Source: CAD feature listing. Evaluate the final solid. Frame: model axes, mm. Give positions to 0.01 mm unless a question says otherwise; leave off trailing zeros. Write each loop counter-clockwise with the first axis right and the second up, starting at its lowest first coordinate (ties: lowest second). Pieces come first, ordered by that corner, then holes. Notation, with made-up numbers: (34.25, 60) - (55.25, 60) arc R20 ccw to (55.25, 68) - close; hole circle Ø4 at (15, -37). An arc over 180 degrees is marked (long way). Answer as a JSON object with one key per item and string values. Group by question number.
from build123d import *

# Parameters (mm, degrees)
SKETCH1_W           = 304.8
SKETCH1_H           = 50.8
SKETCH1_W_2         = 5.9944
SKETCH1_H_2         = 12.7
BOSS_EXTRUDE1_DEPTH = 5.9944
SKETCH3_W           = 247.65
SKETCH3_H           = 1.4875
CUT_EXTRUDE3_DEPTH  = 6.9944
FILLET4_R           = 0.7
SKETCH4_W           = 28.575
SKETCH4_H           = 50.8
BOSS_EXTRUDE2_DEPTH = 5.9944
SKETCH5_W           = 5.9944
SKETCH5_H           = 12.7
CUT_EXTRUDE4_DEPTH  = 6.9944
FILLET5_R           = 3.175
CUT_EXTRUDE5_DEPTH  = 6.9944
CUT_EXTRUDE6_DEPTH  = 6.9944


with BuildPart() as part:
    # Sketch1 → Boss-Extrude1 (new body)
    with BuildSketch(Plane.XY):
        with Locations((-152.4, 25.4)):
            Rectangle(SKETCH1_W, SKETCH1_H)
        with Locations((-15.6972, 12.7)):
            Rectangle(SKETCH1_W_2, SKETCH1_H_2, mode=Mode.SUBTRACT)
        with Locations((-15.6972, 38.1)):
            Rectangle(SKETCH1_W_2, SKETCH1_H_2, mode=Mode.SUBTRACT)
        with Locations((-257.3528, 38.1)):
            Rectangle(SKETCH1_W_2, SKETCH1_H_2, mode=Mode.SUBTRACT)
        with Locations((-257.3528, 12.7)):
            Rectangle(SKETCH1_W_2, SKETCH1_H_2, mode=Mode.SUBTRACT)
        with Locations((-295.4528, 12.7)):
            Rectangle(SKETCH1_W_2, SKETCH1_H_2, mode=Mode.SUBTRACT)
        with Locations((-295.4528, 38.1)):
            Rectangle(SKETCH1_W_2, SKETCH1_H_2, mode=Mode.SUBTRACT)
    extrude(amount=BOSS_EXTRUDE1_DEPTH)

    # Sketch3 → Cut-Extrude3 (cut, through all)
    with BuildSketch(Plane.XY.offset(5.9944)):
        with Locations((-136.525, 50.05625)):
            Rectangle(SKETCH3_W, SKETCH3_H)
        with Locations((-136.525, 0.74375)):
            Rectangle(SKETCH3_W, SKETCH3_H)
    extrude(amount=-CUT_EXTRUDE3_DEPTH, mode=Mode.SUBTRACT)

    # Fillet4
    fillet4_edges = [part.edges().sort_by_distance(p)[0] for p in [
        (-260.35, 49.3125, 2.9972),
        (-260.35, 50.8, 2.9972),
        (-12.7, 50.8, 2.9972),
        (-12.7, 49.3125, 2.9972),
        (-12.7, 0, 2.9972),
        (-260.35, 0, 2.9972),
        (-260.35, 1.4875, 2.9972),
        (-12.7, 1.4875, 2.9972),
    ]]
    fillet(fillet4_edges, radius=FILLET4_R)

    # Sketch4 → Boss-Extrude2 (add)
    with BuildSketch(Plane.XY.offset(5.9944)):
        with Locations((14.2875, 25.4)):
            Rectangle(SKETCH4_W, SKETCH4_H)
    extrude(amount=-BOSS_EXTRUDE2_DEPTH)

    # Sketch5 → Cut-Extrude4 (cut, through all)
    with BuildSketch(Plane.XY.offset(5.9944)):
        with Locations((21.893276, 38.1)):
            Rectangle(SKETCH5_W, SKETCH5_H)
        with Locations((21.893276, 12.7)):
            Rectangle(SKETCH5_W, SKETCH5_H)
    extrude(amount=-CUT_EXTRUDE4_DEPTH, mode=Mode.SUBTRACT)

    # Fillet5
    fillet5_edges = [part.edges().sort_by_distance(p)[0] for p in [
        (28.575, 50.8, 2.9972),
        (28.575, 0, 2.9972),
        (-304.8, 0, 2.9972),
        (-304.8, 50.8, 2.9972),
    ]]
    fillet(fillet5_edges, radius=FILLET5_R)

    # Sketch6 → Cut-Extrude5 (cut, through all)
    with BuildSketch(Plane.XY.offset(5.9944)):
        with BuildLine():
            Line((-123.825, 19.05), (-149.225, 19.05))
            ThreePointArc((-149.225, 19.05), (-155.575, 25.4), (-149.225, 31.75))
            Line((-149.225, 31.75), (-123.825, 31.75))
            ThreePointArc((-123.825, 31.75), (-117.475, 25.4), (-123.825, 19.05))
        make_face()
        with BuildLine():
            Line((-60.325, 19.05), (-85.725, 19.05))
            ThreePointArc((-85.725, 19.05), (-92.075, 25.4), (-85.725, 31.75))
            Line((-85.725, 31.75), (-60.325, 31.75))
            ThreePointArc((-60.325, 31.75), (-53.975, 25.4), (-60.325, 19.05))
        make_face()
        with BuildLine():
            Line((-187.325, 19.05), (-212.725, 19.05))
            ThreePointArc((-212.725, 19.05), (-219.075, 25.4), (-212.725, 31.75))
            Line((-212.725, 31.75), (-187.325, 31.75))
            ThreePointArc((-187.325, 31.75), (-180.975, 25.4), (-187.325, 19.05))
        make_face()
    extrude(amount=-CUT_EXTRUDE5_DEPTH, mode=Mode.SUBTRACT)

    # Sketch7 → Cut-Extrude6 (cut, through all)
    with BuildSketch(Plane.XY.offset(5.9944)):
        with BuildLine():
            Line((-6.35, 12.7), (-6.35, 38.1))
            ThreePointArc((-6.35, 38.1), (-4.7625, 39.6875), (-3.175, 38.1))
            Line((-3.175, 38.1), (-3.175, 12.7))
            ThreePointArc((-3.175, 12.7), (-4.7625, 11.1125), (-6.35, 12.7))
        make_face()
        with BuildLine():
            Line((1.524, 12.7), (1.524, 38.1))
            ThreePointArc((1.524, 38.1), (3.1115, 39.6875), (4.699, 38.1))
            Line((4.699, 38.1), (4.699, 12.7))
            ThreePointArc((4.699, 12.7), (3.1115, 11.1125), (1.524, 12.7))
        make_face()
        with BuildLine():
            Line((9.398, 12.7), (9.398, 38.1))
            ThreePointArc((9.398, 38.1), (10.9855, 39.6875), (12.573, 38.1))
            Line((12.573, 38.1), (12.573, 12.7))
            ThreePointArc((12.573, 12.7), (10.9855, 11.1125), (9.398, 12.7))
        make_face()
    extrude(amount=-CUT_EXTRUDE6_DEPTH, mode=Mode.SUBTRACT)


solid = part.part
Q1. Ray query, probe 1 along X at (y, z) = (7, 1.75) (3 decimals); probe 2 along Y at (x, z) = (-138, 5.25); probe 3 along Y at (x, z) = (-86, 4.25). Return the intervals inside material, ascending. Write a range as [from, to].
Q2. Section B-B on z = 4.15. State how many separate pieces and enclosed holes the cut face has, then the cut area to 3 significant figures.
Q3. First-contact query: pin 1 Ø2 at (x, z) = (-80.5, 5) entering from -Y; pin 2 Ø5 at (x, y) = (-40.5, 26.5) entering from -Z; pin 3 Ø3 at (x, z) = (-135.5, 2) entering from +Y. Flat tips, straight axial feed; report the tip coordinate or a pass-through.
Q4. Draft query along Y for faces 1 (the flat face through (-140, 14, 5.994)), 2 (the flat face through (-12.7, 38, 3)). Return one class per face: released by +Y, released by -Y, zero draft, split by the parting line, or undercut.
Q5. Section C-C on x = -108. Return the cut outline in (y, z), then the cut area to 3 significant figures.
Q6. Section A-A on y = 25.4. Return the cut outline in (x, z) (3 decimals), then the cut area to 3 significant figures.
Taken from the geometry:
{
 "1": {"probe 1": "x = [-304.8, -298.45], [-292.456, -260.35], [-254.356, -18.694], [-12.7, 18.896], [24.89, 28.575]", "probe 2": "y = [1.49, 19.05], [31.75, 49.31]", "probe 3": "y = [1.49, 19.06], [31.74, 49.31]"},
 "2": {"separate pieces": "1", "enclosed holes": "14", "area": "14,000 mm²"},
 "3": {"pin 1": "stops at y = 1.49", "pin 2": "stops at z = 0", "pin 3": "stops at y = 49.31"},
 "4": {"face 1": "zero draft", "face 2": "undercut"},
 "5": {"outline": "(1.49, 0) - (49.31, 0) - (49.31, 5.99) - (1.49, 5.99) - close", "area": "287 mm²"},
 "6": {"outline": "(-304.8, 0) - (-219.075, 0) - (-219.075, 5.994) - (-304.8, 5.994) - close; (-180.975, 0) - (-155.575, 0) - (-155.575, 5.994) - (-180.975, 5.994) - close; (-117.475, 0) - (-92.075, 0) - (-92.075, 5.994) - (-117.475, 5.994) - close; (-53.975, 0) - (-6.35, 0) - (-6.35, 5.994) - (-53.975, 5.994) - close; (-3.175, 0) - (1.524, 0) - (1.524, 5.994) - (-3.175, 5.994) - close; (4.699, 0) - (9.398, 0) - (9.398, 5.994) - (4.699, 5.994) - close; (12.573, 0) - (28.575, 0) - (28.575, 5.994) - (12.573, 5.994) - close", "area": "1,260 mm²"}
}
